Verification items for this drawing (mm, ordinates from the low corner). A direction names the side the tool comes from. Round coordinates to 2 decimals unless told otherwise and drop trailing zeros. Order: outer loops, then holes, each group sorted by start corner. A loop starts at its lowest first (then second) coordinate and runs counter-clockwise, first axis right, second up.
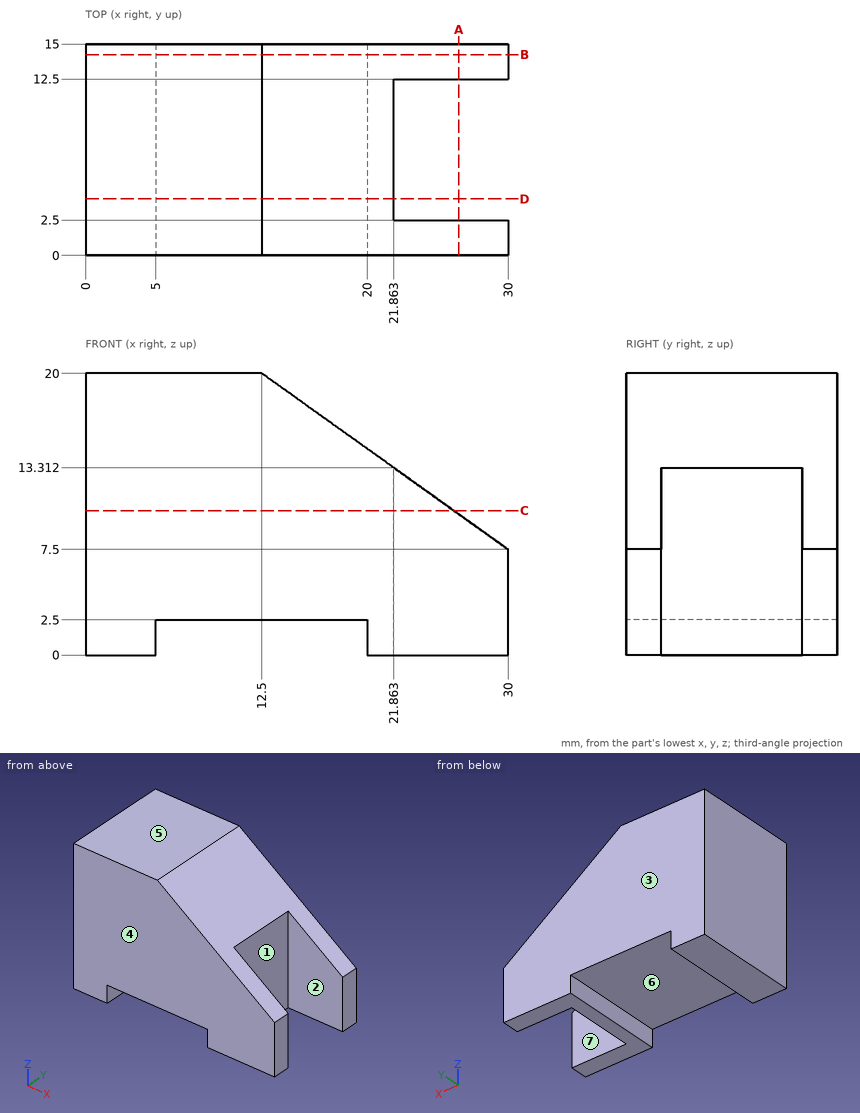
Item 1: Release check for a two-part mould opening along Y. For the marked faces 1, 2, 3 and 4 record: released by +Y, released by -Y, zero draft, split by the parting line, or undercut.
Answer:
face 1: undercut
face 2: undercut
face 3: released by +Y
face 4: released by -Y
Item 2: Sectioned sample at A-A (x = 26.5). Record the cut outline in (y, z).
Answer:
outline: (0, 0) - (2.5, 0) - (2.5, 10) - (0, 10) - close; (12.5, 0) - (15, 0) - (15, 10) - (12.5, 10) - close
Item 3: Go/stop test with flat-tipped pins: P1, Ø5, axis at y = 6, z = 8, coming from the +X side; P2, Ø3, axis at x = 25, z = 13, coming from the +Y side. Record where each tip stops, or that it passes through.
Answer:
P1: stops at x = 21.86
P2: passes through
Item 4: Sectioned sample at B-B (y = 14.25). Record the cut outline in (x, z), and give its area (3 significant figures).
Answer:
outline: (0, 0) - (5, 0) - (5, 2.5) - (20, 2.5) - (20, 0) - (30, 0) - (30, 7.5) - (12.5, 20) - (0, 20) - close
area: 453 mm2
Item 5: Sectioned sample at D-D (y = 4). Record the cut outline in (x, z).
Answer:
outline: (0, 0) - (5, 0) - (5, 2.5) - (20, 2.5) - (20, 0) - (21.86, 0) - (21.86, 13.31) - (12.5, 20) - (0, 20) - close
Item 6: Scan lines: line 1 along X through (y, z) = (7.5, 9.75); line 2 along Z through (x, y) = (8.5, 5); line 3 along X through (y, z) = (9.25, 15.75). Record each from-to range of solid material in increasing order.
Answer:
line 1: x = 0 to 21.86
line 2: z = 2.5 to 20
line 3: x = 0 to 18.45
Item 7: Sectioned sample at C-C (z = 10.25). Record the cut outline in (x, y), and give its area (3 significant figures).
Answer:
outline: (0, 0) - (26.15, 0) - (26.15, 2.5) - (21.86, 2.5) - (21.86, 12.5) - (26.15, 12.5) - (26.15, 15) - (0, 15) - close
area: 349 mm2
Item 8: Access from +Z, -Z, +X, -X, +Y, -Y to the whole of each face (thin tool, end or side, straight path). Record for the marked faces 5, 6 and 7.
Answer:
face 5: +Z, +X, -X, +Y, -Y
face 6: -Z, +Y, -Y
face 7: +Z, -Z, +X
